Could you check a few things on this model? Use its own coordinates, in mm. A direction names the side the tool comes from. Coordinates: 2 decimals unless noted, no trailing zeros. Write each loop counter-clockwise with the first axis right and the second up, starting at its lowest first coordinate (ties: lowest second). Pieces come first, ordered by that corner, then holes. Notation, with made-up numbers: M -25,89.5 L 8,89.5 A22 cw 8,104.5 Z; hole C 3.25,19 d9. An arc over 180 degrees is marked long. Write item = value, one per line.
```python
from build123d import *

# Parameters (mm, degrees)
SKETCH1_W                 = 134.82228219
SKETCH1_H                 = 4.73075
CHAMFER1_SIZE             = 0.508
F_8_32_TAPPED_HOLE1_D     = 3.4544
F_8_32_TAPPED_HOLE1_DEPTH = 10.7188
F_8_32_TAPPED_HOLE1_TIP   = 1.037806461
F_8_32_TAPPED_HOLE3_D     = 3.4544
F_8_32_TAPPED_HOLE3_DEPTH = 10.7188
F_8_32_TAPPED_HOLE3_TIP   = 1.037806461


with BuildPart() as part:
    # Sketch1 → Revolve1 (revolve)
    with BuildSketch(Plane(origin=(0, 0, 0), x_dir=(0, 0, -1), z_dir=(1, 0, 0)), mode=Mode.PRIVATE) as revolve1_sk:
        with Locations((67.411141095, 2.365375)):
            Rectangle(SKETCH1_W, SKETCH1_H)
    revolve(revolve1_sk.sketch.rotate(Axis((0, 0, 0), (0, 0, 1)), 90), axis=Axis((0, 0, 0), (0, 0, 1)))

    # Chamfer1
    chamfer1_edges = [part.edges().sort_by_distance(p)[0] for p in [
        (4.73075, 0, -134.82228219),
        (4.73075, 0, 0),
    ]]
    chamfer(chamfer1_edges, length=CHAMFER1_SIZE)

    # #8-32 Tapped Hole1
    with Locations(Plane.XY):
        with Locations((0, 0)):
            Hole(F_8_32_TAPPED_HOLE1_D / 2, depth=F_8_32_TAPPED_HOLE1_DEPTH)
            with Locations((0, 0, -(F_8_32_TAPPED_HOLE1_DEPTH + F_8_32_TAPPED_HOLE1_TIP / 2))):  # 118° drill point
                Cone(0, F_8_32_TAPPED_HOLE1_D / 2, F_8_32_TAPPED_HOLE1_TIP, mode=Mode.SUBTRACT)

    # #8-32 Tapped Hole3
    with Locations(Plane(origin=(0, 0, -134.82228219), x_dir=(-1, 0, 0), z_dir=(0, 0, -1))):
        with Locations((0, 0)):
            Hole(F_8_32_TAPPED_HOLE3_D / 2, depth=F_8_32_TAPPED_HOLE3_DEPTH)
            with Locations((0, 0, -(F_8_32_TAPPED_HOLE3_DEPTH + F_8_32_TAPPED_HOLE3_TIP / 2))):  # 118° drill point
                Cone(0, F_8_32_TAPPED_HOLE3_D / 2, F_8_32_TAPPED_HOLE3_TIP, mode=Mode.SUBTRACT)


solid = part.part
```
Item 1: I'm going to push flat-ended pins straight in: P1, Ø2, axis at x = 0, y = 0, coming from the +Z side; P2, Ø2, axis at y = 1.5, z = -80.5, coming from the +X side; P3, Ø1.5, axis at x = -2, z = -60.5, coming from the -Y side. Where does each tip first touch, or does it pass through?
Numbers:
P1 = -11.16
P2 = 4.7
P3 = -4.56
Item 2: If I drill on line 1 along Y through (x, z) = (0, -128.25); line 2 along X through (y, z) = (0.25, -129); line 3 along X through (y, z) = (0.5, -119.5), over which ranges is the centre line in solid material (lowest first)?
Numbers:
line_1 = -4.73 to -1.73, 1.73 to 4.73
line_2 = -4.72 to -1.71, 1.71 to 4.72
line_3 = -4.7 to 4.7
Item 3: Imagine slicing it at B-B (z = -30). Write out the boundary of the cut face in (x, y), and give its area (3 significant figures).
Numbers:
outline = C 0,0 d9.46
area = 70.3 mm²
Item 4: For faces 4 (the face through (0.225, 1.713, -5.434)), 5 (the face through (0, 2, 0)), which set-ups out of +Z, -Z, +X, -X, +Y, -Y let a thin tool reach every point of the face, with its end or its side?
Numbers:
face_4 = +Z
face_5 = +Z, +X, -X, +Y, -Y
Item 5: Imagine slicing it at A-A (z = -9.5). Write out the boundary of the cut face in (x, y), and give its area (3 significant figures).
Numbers:
outline = C 0,0 d9.46; hole C 0,0 d3.45
area = 60.9 mm²
Item 6: If we mould it in two halves opening along Y, with no side actions, what happens to faces 1 (the face through (0, 2, -134.822)), 2 (the face through (-0.225, 1.713, -129.388)), 3 (the face through (-4.512, -1.421, -68.348))? For each: pulls with the +Y half, pulls with the -Y half, needs draft (parallel to the pull), parting line crosses it, or undercut.
Numbers:
face_1 = needs draft
face_2 = undercut
face_3 = parting line crosses it
